```python
from build123d import *

# Parameters (mm, degrees)
F1_DEPTH = 25
F2_T     = -2.5


with BuildPart() as f1:
    # F0 (on Top) → F1 (new body)
    with BuildSketch(Plane.XY):
        Polygon((36.507031, 48.091673), (-43.492969, 48.091673), (-32.188456, 0), (36.507031, 0), align=None)
    extrude(amount=F1_DEPTH)

    # F2
    f2_openings = [f1.faces().sort_by_distance(p)[0] for p in [
        (-0.738459, 24.655195, 25),
    ]]
    offset(amount=F2_T, openings=f2_openings)


solid = f1.part
```
Model file for the job. Use its own axes, mm. A direction names the side the tool comes from. Round coordinates to 2 decimals unless told otherwise and drop trailing zeros. Order: outer loops, then holes, each group sorted by start corner. A loop starts at its lowest first (then second) coordinate and runs counter-clockwise, first axis right, second up. Notation, with made-up numbers: M -9,50.25 L 37,50.25 A36 ccw 37,88.25 Z; hole C 28.5,37.5 d4. An arc over 180 degrees is marked long. Use CSV: the item, a comma, the result in double quotes.
Item 1: Saw through at B-B (x = 25). List the corners of the cut face in (y, z).
Worked answers:
outline,"M 0,0 L 48.09,0 L 48.09,25 L 45.59,25 L 45.59,2.5 L 2.5,2.5 L 2.5,25 L 0,25 Z"
Item 2: Pin check, flat tips, straight feed: pin 1 (2 mm diameter, centred on y = 24.5, z = 14, fed in from -X); pin 2 (4 mm diameter, centred on y = 18, z = 13.5, fed in from -X); pin 3 (11 mm diameter, centred on y = 26, z = 8.5, fed in from -X). Stop position of each tip, or through.
Worked answers:
pin 1,"x = -38.18"
pin 2,"x = -36.89"
pin 3,"x = -39.59"
Item 3: Probe probe 1 along Y at (x, z) = (-29.5, 15.5); probe 2 along Z at (x, y) = (-25, 33); probe 3 along X at (y, z) = (9.5, 6.5). List the from-to ranges inside material, lowest first.
Worked answers:
probe 1,"0 to 2.5, 45.59 to 48.09"
probe 2,"0 to 2.5"
probe 3,"-34.42 to -31.85, 34.01 to 36.51"
Item 4: Saw through at C-C (y = 29.5). List the corners of the cut face in (x, z).
Worked answers:
outline,"M -39.12,0 L 36.51,0 L 36.51,25 L 34.01,25 L 34.01,2.5 L -36.55,2.5 L -36.55,25 L -39.12,25 Z"
Item 5: Pull direction Y, two halves, no side cores. Call faces 1 (the face through (-37.92, 24.38, 12.32)), 2 (the face through (-1, 47, 25)), 3 (the face through (1, 2.5, 14)): released by +Y, released by -Y, zero draft, split by the parting line, or undercut.
Worked answers:
face 1,"released by -Y"
face 2,"zero draft"
face 3,"undercut"
Item 6: Saw through at A-A (z = 17). List the corners of the cut face in (x, y).
Worked answers:
outline,"M -43.49,48.09 L -32.19,0 L 36.51,0 L 36.51,48.09 Z; hole M -40.34,45.59 L -30.21,2.5 L 34.01,2.5 L 34.01,45.59 Z"
Item 7: Which spindle directions (+Z, -Z, +X, -X, +Y, -Y) get a long thin tool onto all of the face, cutting with end or side? Do faces 4 (the face through (-3, 48.092, 12)), 5 (the face through (-4, 24, 2.5)). Say none if no direction does.
Worked answers:
face 4,"+Z, -Z, +X, -X, +Y"
face 5,"+Z"
